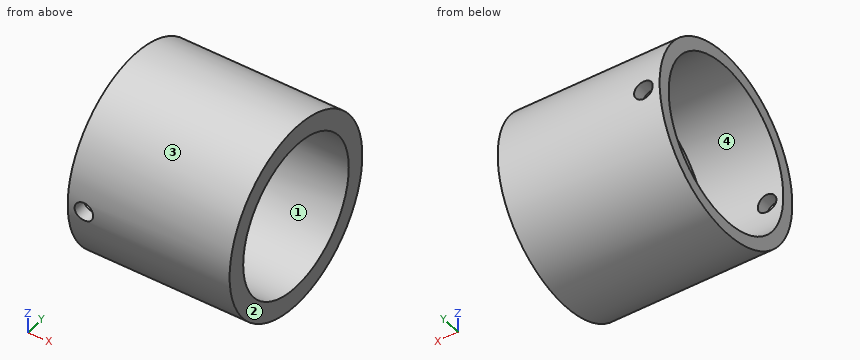
```python
from build123d import *

# Parameters (mm, degrees)
CROQUIS4_R                 = 1.435
CORTAR_EXTRUIR1_DEPTH      = 15.675
CORTAR_EXTRUIR1_DEPTH_BACK = 15.675


with BuildPart() as part:
    # Croquis3 → Revolución1 (revolve)
    with BuildSketch(Plane(origin=(0, 0, 0), x_dir=(1, 0, 0), z_dir=(0, 1, 0))):
        Polygon((0, 11.675), (-13, 11.675), (-13, 12.675), (-25, 12.675), (-25, 14.675), (0, 14.675), align=None)
    revolve(axis=Axis((-30.367380332, 0, 0), (1, 0, 0)))

    # Croquis4 → Cortar-Extruir1 (cut, two sides)
    with BuildSketch(Plane(origin=(0, 0, 0), x_dir=(1, 0, 0), z_dir=(0, 1, 0))) as cortar_extruir1_sk:
        with Locations((-22.5, 0)):
            Circle(CROQUIS4_R)
    extrude(amount=CORTAR_EXTRUIR1_DEPTH, mode=Mode.SUBTRACT)
    extrude(cortar_extruir1_sk.sketch, amount=-CORTAR_EXTRUIR1_DEPTH_BACK, mode=Mode.SUBTRACT)


solid = part.part
```
Model file for the job. Use its own axes, mm. Face numbers are marked on the shaded views. Give positions to 0.01 mm unless a question says otherwise; leave off trailing zeros. Order: outer loops, then holes, each group sorted by start corner. A loop starts at its lowest first (then second) coordinate and runs counter-clockwise, first axis right, second up.
1) Wall check: probe 1 along Y at (x, z) = (-10.5, 0) (3 decimals); probe 2 along X at (y, z) = (-14.05, 0) (3 decimals); probe 3 along Z at (x, y) = (-17.25, -0.25). Give the ranges that are in metal, low to high.
2) Saw through at D-D, the plane x = -10.75. Write the cut outline in (y, z) (3 decimals).
3) Mould opens along Y. For the marked faces 1, 2, 3 and 4 say: +Y half, -Y half, draft (parallel to the pull), parting line (faces both ways), or undercut.
4) Pin check, flat tips, straight feed: pin 1 (1 mm diameter, centred on x = -7.5, z = 6.5, fed in from +Y); pin 2 (5 mm diameter, centred on x = -13.5, z = 4, fed in from -Y); pin 3 (5 mm diameter, centred on x = -9.5, y = -10, fed in from -Z). Stop position of each tip, or through.
5) Saw through at A-A, the plane y = 0. Write the cut outline in (x, z) (3 decimals).
6) Saw through at C-C, the plane z = 7.5. Write the cut outline in (x, y).
7) Saw through at B-B, the plane z = 0. Write the cut outline in (x, y) (3 decimals), then the cut area to 3 significant figures.
Computed:
1. probe 1: y = -14.675 to -11.675, 11.675 to 14.675
1. probe 2: x = -25 to -23.935, -21.065 to 0
1. probe 3: z = -14.67 to -12.67, 12.67 to 14.67
2. outline: circle Ø29.35 at (0, 0); hole circle Ø23.35 at (0, 0)
3. face 1: undercut
3. face 2: draft
3. face 3: parting line
3. face 4: undercut
4. pin 1: stops at y = 13.39
4. pin 2: stops at y = -14.6
4. pin 3: stops at z = -12.61
5. outline: (-25, -14.675) - (0, -14.675) - (0, -11.675) - (-13, -11.675) - (-13, -12.675) - (-25, -12.675) - close; (-25, 12.675) - (-13, 12.675) - (-13, 11.675) - (0, 11.675) - (0, 14.675) - (-25, 14.675) - close
6. outline: (-25, -12.61) - (0, -12.61) - (0, -8.95) - (-13, -8.95) - (-13, -10.22) - (-25, -10.22) - close; (-25, 10.22) - (-13, 10.22) - (-13, 8.95) - (0, 8.95) - (0, 12.61) - (-25, 12.61) - close
7. outline: (-25, -14.675) - (-23.935, -14.675) - (-23.935, -12.675) - (-25, -12.675) - close; (-25, 12.675) - (-23.935, 12.675) - (-23.935, 14.675) - (-25, 14.675) - close; (-21.065, -14.675) - (0, -14.675) - (0, -11.675) - (-13, -11.675) - (-13, -12.675) - (-21.065, -12.675) - close; (-21.065, 12.675) - (-13, 12.675) - (-13, 11.675) - (0, 11.675) - (0, 14.675) - (-21.065, 14.675) - close
7. area: 115 mm2
